from build123d import *
from build123d.topology import SkipClean

# Parameters (mm, degrees)
SKETCH1_R           = 1.6
BOSS_EXTRUDE1_DEPTH = 12.7
SKETCH2_W           = 48.3
SKETCH2_H           = 8
BOSS_EXTRUDE2_DEPTH = 12.7
CUT_EXTRUDE3_DEPTH  = 73.098404975
FILLET1_R           = 3.175


with BuildPart() as part:
    # Sketch1 → Boss-Extrude1 (new body)
    with BuildSketch(Plane.XY):
        with BuildLine():
            Line((48.3, 0), (0, 0))
            Line((0, 0), (0, -18.258342613))
            ThreePointArc((0, -18.258342613), (4.621320344, -18.031373033), (7, -22))
            ThreePointArc((7, -22), (4.621320344, -25.968626967), (0, -25.741657387))
            Line((0, -25.741657387), (0, -44))
            Line((0, -44), (48.3, -44))
            Line((48.3, -44), (48.3, 0))
        make_face()
        with Locations((7.5, -37)):
            Circle(SKETCH1_R, mode=Mode.SUBTRACT)
        with Locations((37.5, -37)):
            Circle(SKETCH1_R, mode=Mode.SUBTRACT)
        with Locations((7.5, -7)):
            Circle(SKETCH1_R, mode=Mode.SUBTRACT)
        with Locations((37.5, -7)):
            Circle(SKETCH1_R, mode=Mode.SUBTRACT)
    extrude(amount=BOSS_EXTRUDE1_DEPTH)

    # Sketch2 → Boss-Extrude2 (add)
    with BuildSketch(Plane.XY.offset(12.7)):
        Polygon((0, -52), (0, -44), (0, -25.741657387), (0, -18.258342613), (0, 0), (-5, 0), (-5, -52), align=None)
        with Locations((24.15, -48)):
            Rectangle(SKETCH2_W, SKETCH2_H)
    extrude(amount=-BOSS_EXTRUDE2_DEPTH)

    # Sketch1<5> → Cut-Extrude3 (cut, through all)
    with SkipClean():  # the faces are left unmerged after this step: merging them gives an invalid solid
        with BuildSketch(Plane.XY):
            with BuildLine():
                ThreePointArc((7, -22), (4.621320344, -18.031373033), (0, -18.258342613))
                Line((0, -18.258342613), (0, -25.741657387))
                ThreePointArc((0, -25.741657387), (4.621320344, -25.968626967), (7, -22))
            make_face()
            with BuildLine():
                Line((0, -25.741657387), (0, -18.258342613))
                ThreePointArc((0, -18.258342613), (-2, -22), (0, -25.741657387))
            make_face()
        extrude(amount=CUT_EXTRUDE3_DEPTH, mode=Mode.SUBTRACT)

    # Fillet1
    fillet1_edges = [part.edges().sort_by_distance(p)[0] for p in [
        (48.3, 0, 6.35),
        (-5, 0, 6.35),
        (48.3, -52, 6.35),
        (-5, -52, 6.35),
    ]]
    fillet(fillet1_edges, radius=FILLET1_R)


solid = part.part
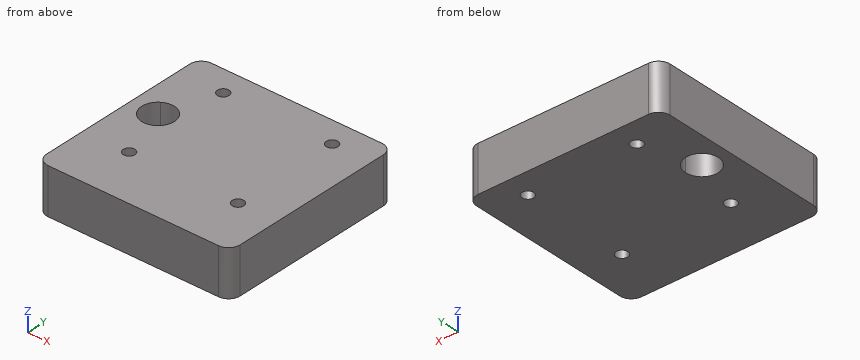
Could you check a few things on this model? Use its own coordinates, in mm. Round coordinates to 2 decimals unless told otherwise and drop trailing zeros. Order: outer loops, then holes, each group sorted by start corner. A loop starts at its lowest first (then second) coordinate and runs counter-clockwise, first axis right, second up.
Q1. Imagine slicing it at B-B, the plane z = 5.25. List the corners of the cut face in (x, y) for me (3 decimals).
Geometry says:
outline: (-5, -48.825) arc R3.175 ccw to (-1.825, -52) - (45.125, -52) arc R3.175 ccw to (48.3, -48.825) - (48.3, -3.175) arc R3.175 ccw to (45.125, 0) - (-1.825, 0) arc R3.175 ccw to (-5, -3.175) - close; hole circle Ø9 at (2.5, -22); hole circle Ø3.2 at (7.5, -37); hole circle Ø3.2 at (7.5, -7); hole circle Ø3.2 at (37.5, -37); hole circle Ø3.2 at (37.5, -7)
Q2. Please list where these lines run through material, in increasing order: probe 1 along Y at (x, z) = (7.5, 4); probe 2 along X at (y, z) = (-8, 8.75); probe 3 along Y at (x, z) = (38, 9.25).
Geometry says:
probe 1: y = -52 to -38.6, -35.4 to -8.6, -5.4 to 0
probe 2: x = -5 to 6.25, 8.75 to 36.25, 38.75 to 48.3
probe 3: y = -52 to -38.52, -35.48 to -8.52, -5.48 to 0
Q3. Imagine slicing it at C-C, the plane y = -37. List the corners of the cut face in (x, z) for me, then the cut area to 3 significant figures.
Geometry says:
outline: (-5, 0) - (5.9, 0) - (5.9, 12.7) - (-5, 12.7) - close; (9.1, 0) - (35.9, 0) - (35.9, 12.7) - (9.1, 12.7) - close; (39.1, 0) - (48.3, 0) - (48.3, 12.7) - (39.1, 12.7) - close
area: 596 mm2
Q4. Imagine slicing it at A-A, the plane x = 37.5. List the corners of the cut face in (y, z) for me, then the cut area to 3 significant figures.
Geometry says:
outline: (-52, 0) - (-38.6, 0) - (-38.6, 12.7) - (-52, 12.7) - close; (-35.4, 0) - (-8.6, 0) - (-8.6, 12.7) - (-35.4, 12.7) - close; (-5.4, 0) - (0, 0) - (0, 12.7) - (-5.4, 12.7) - close
area: 579 mm2
